Autodesk Inventor part; units mm, degrees
ref_plane "YZ Plane" through (0, 0, 0) normal (1, 0, 0) x (0, 1, 0)
ref_plane "XZ Plane" through (0, 0, 0) normal (0, 1, 0) x (-1, 0, 0)
ref_plane "XY Plane" through (0, 0, 0) normal (0, 0, 1) x (1, 0, 0)
sketch "Sketch1" plane through (0, 0, 0) normal (0, 0, 1) x (1, 0, 0)
  circle A0 centre (0, 0) radius 7.5
  line L0 (11.4997, 8) -> (8.4997, 8)
  line L1 (8.4997, 8) -> (8.4997, 12)
  line L2 (8.4997, -12) -> (8.4997, -8)
  line L3 (8.4997, -8) -> (11.4997, -8)
  line L4 (-10.667, -15) -> (-10.667, -12)
  line L5 (-10.667, -12) -> (-14.5003, -12)
  line L6 (4.6663, -15) -> (4.6663, -12)
  line L7 (4.6663, -12) -> (8.4997, -12)
  line L8 (-17.5003, -8) -> (-14.5003, -8)
  line L9 (-14.5003, -8) -> (-14.5003, -12)
  line L10 (-17.5003, 8) -> (-14.5003, 8)
  line L11 (-14.5003, 8) -> (-14.5003, 12)
  line L12 (-10.667, 15) -> (-10.667, 12)
  line L13 (-10.667, 12) -> (-14.5003, 12)
  line L14 (8.4997, 12) -> (4.6663, 12)
  line L15 (4.6663, 12) -> (4.6663, 15)
  line L16 (11.4997, 8) -> (11.4997, -8)
  line L17 (-10.667, 15) -> (4.6663, 15)
  line L18 (-17.5003, -8) -> (-17.5003, 8)
  line L19 (4.6663, -15) -> (-10.667, -15)
  line L20 (11.4997, -7) -> (11.4997, 8)
  line L21 (-20.9424, 0) -> (31.3224, 0) construction
  line L22 (-0.0003, 36) -> (-0.0003, -23) construction
  dimension "d0" = 15
  dimension "d3" = 3
  dimension "d5" = 3
  dimension "d6" = 3
  dimension "d15" = 30
  dimension "d16" = 3
  dimension "d22" = 8.5
  dimension "d23" = 14.5
  dimension "d24" = 23
  dimension "d25" = 15.3333
  dimension "d26" = 24
  dimension "d27" = 16
extrude "Extrusion1" add sketch "Sketch1" along normal mid plane 3
equation "\"d25\" = 0.666667 * d24"
equation "\"d27\" = 0.666667 * d26"
properties part number "Camera-Holder_Bearing-Ring-Middle-Left"
The listing builds one solid part. Answer for the finished solid, in the listing's coordinates (mm). A direction names the side the tool comes from. Give positions to 0.01 mm unless a question says otherwise; leave off trailing zeros. Write each loop counter-clockwise with the first axis right and the second up, starting at its lowest first coordinate (ties: lowest second). Pieces come first, ordered by that corner, then holes. Notation, with made-up numbers: (29.5, -5) -> (82.5, -5) arc R30 cw to (82.5, 17) -> close; hole circle Ø7 at (20.25, 9). An arc over 180 degrees is marked (long way). Write item = value, one per line. Start each with the question number.
1) The part is cut by section C-C, the plane z = 0.5. Determine the outline of the cut face in (x, y), and give its area (3 significant figures).
2) The part is cut by section A-A, the plane y = 0. Determine the outline of the cut face in (x, z).
3) Determine the mould class of faces 1 (the face through (7, 12, 0)), 2 (the face through (-7.493, -0.33, -0.021)), 3 (the face through (8.5, -10, 0)), 4 (the face through (-3, -15, 0)) for opening direction Y: +Y half, -Y half, draft (parallel to the pull), parting line (faces both ways), or undercut.
4) Straight lines are drawn through the part: line 1 along Y through (x, z) = (0, 0.45); line 2 along X through (y, z) = (-12.25, 0.4); line 3 along Y through (x, z) = (-12, 0.15). For each, find the intervals that lie inside material, in ascending order.
5) Each of these flat-tipped pins is pushed along its axis until it touches: pin 1 (1.5 mm diameter, centred on y = -10, z = 0, fed in from +X); pin 2 (0.9 mm diameter, centred on y = -13.5, z = -0.5, fed in from +X); pin 3 (0.9 mm diameter, centred on x = -12.5, z = -0.5, fed in from -Y). Where does it stop, or does it pass through?
6) The part is cut by section D-D, the plane x = -14. Determine the outline of the cut face in (y, z).
7) The part is cut by section B-B, the plane x = 0. Determine the outline of the cut face in (y, z).
8) Which of the six approach directions +Z, -Z, +X, -X, +Y, -Y give full straight-line access (tool end or side, diameter ignored) to faces 5 (the face through (-14.5, 10, 0)), 6 (the face through (4.666, 13, 0)), 7 (the face through (-10.667, -14, 0)), 8 (the face through (10, -8, 0))?
Solutions:
q1.outline = (-17.5, -8) -> (-14.5, -8) -> (-14.5, -12) -> (-10.67, -12) -> (-10.67, -15) -> (4.67, -15) -> (4.67, -12) -> (8.5, -12) -> (8.5, -8) -> (11.5, -8) -> (11.5, 8) -> (8.5, 8) -> (8.5, 12) -> (4.67, 12) -> (4.67, 15) -> (-10.67, 15) -> (-10.67, 12) -> (-14.5, 12) -> (-14.5, 8) -> (-17.5, 8) -> close; hole circle Ø15 at (0, 0)
q1.area = 563 mm²
q2.outline = (-17.5, -1.5) -> (-7.5, -1.5) -> (-7.5, 1.5) -> (-17.5, 1.5) -> close; (7.5, -1.5) -> (11.5, -1.5) -> (11.5, 1.5) -> (7.5, 1.5) -> close
q3.face_1 = +Y half
q3.face_2 = undercut
q3.face_3 = draft
q3.face_4 = -Y half
q4.line_1 = -15 to -7.5, 7.5 to 15
q4.line_2 = -10.67 to 4.67
q4.line_3 = -12 to 12
q5.pin_1 = 8.5
q5.pin_2 = 4.67
q5.pin_3 = -12
q6.outline = (-12, -1.5) -> (12, -1.5) -> (12, 1.5) -> (-12, 1.5) -> close
q7.outline = (-15, -1.5) -> (-7.5, -1.5) -> (-7.5, 1.5) -> (-15, 1.5) -> close; (7.5, -1.5) -> (15, -1.5) -> (15, 1.5) -> (7.5, 1.5) -> close
q8.face_5 = +Z, -Z, -X, +Y
q8.face_6 = +Z, -Z, +X, +Y
q8.face_7 = +Z, -Z, -X, -Y
q8.face_8 = +Z, -Z, +X, -Y
